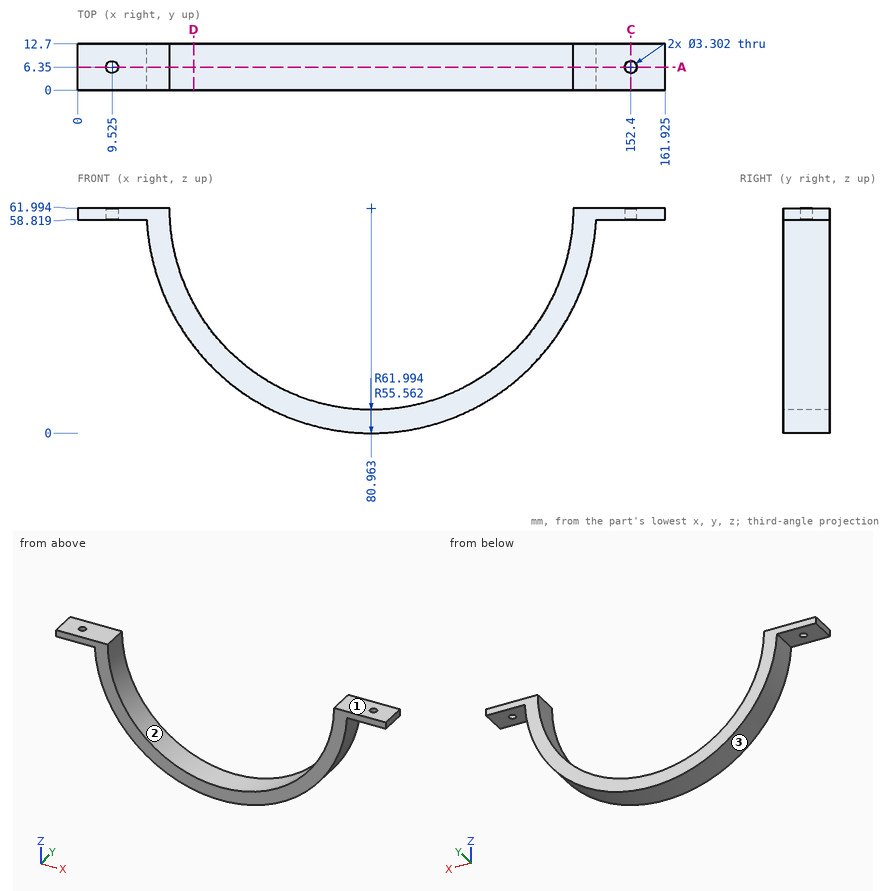
Here's the drawing with two shaded views (mm, measured from the low corner). I have some questions. Give positions to 0.01 mm unless a question says otherwise; leave off trailing zeros. Loops run counter-clockwise (first coordinate to the right, second up) from the corner with the lowest first, then second, coordinate; pieces in that order, holes last. Notation, with made-up numbers: M 16,-9.75 L 35,-9.75 A16 ccw 35,0.25 Z; hole C 22.25,68.25 d10. An arc over 180 degrees is marked long. Answer in a Markdown table with one row per item.
1. If I drill on line 1 along Y through (x, z) = (152.4, 61.3); line 2 along X through (y, z) = (2, 55) (1 decimal); line 3 along X through (y, z) = (10, 57.5), over which ranges is the centre line in solid material (lowest first)?
Taken from the geometry:
| item | result |
|---|---|
| line 1 | y = 0 to 4.7, 8 to 12.7 |
| line 2 | x = 19.4 to 25.8, 136.1 to 142.6 |
| line 3 | x = 19.13 to 25.58, 136.34 to 142.79 |
2. For pin 1 Ø5.5 at (x, y) = (152.4, 6.35) entering from -Z; pin 2 Ø3 at (y, z) = (4, 13) entering from +X (1 decimal); pin 3 Ø10 at (x, z) = (86, 8) entering from +Y; pin 4 Ø1.5 at (y, z) = (8.5, 42) entering from +X, each with a flat end and sliding along its axis, tell me the tip position at first contact or that it passes through.
Taken from the geometry:
| item | result |
|---|---|
| pin 1 | stops at z = 58.82 |
| pin 2 | stops at x = 120.8 |
| pin 3 | stops at y = 12.7 |
| pin 4 | stops at x = 139.89 |
3. Suppose I cut it at C-C on x = 152.4. Write out the boundary of the cut face in (y, z).
Taken from the geometry:
| item | result |
|---|---|
| outline | M 0,58.82 L 4.7,58.82 L 4.7,61.99 L 0,61.99 Z; M 8,58.82 L 12.7,58.82 L 12.7,61.99 L 8,61.99 Z |
4. Suppose I cut it at D-D on x = 32. Write out the boundary of the cut face in (y, z), plus the area to 3 significant figures.
Taken from the geometry:
| item | result |
|---|---|
| outline | M 0,23.97 L 12.7,23.97 L 12.7,35.73 L 0,35.73 Z |
| area | 149 mm² |
5. Thinking about a two-plate mould opening in X: for the marked faces 1, 2 and 3, which applies, released by +X, released by -X, zero draft, split by the parting line, or undercut?
Taken from the geometry:
| item | result |
|---|---|
| face 1 | zero draft |
| face 2 | undercut |
| face 3 | split by the parting line |
6. Suppose I cut it at A-A on y = 6.35. Count the separate pieces of the cut face and the enclosed holes in it, plus the area to 3 significant figures.
Taken from the geometry:
| item | result |
|---|---|
| separate pieces | 3 |
| enclosed holes | 0 |
| area | 1,290 mm² |
